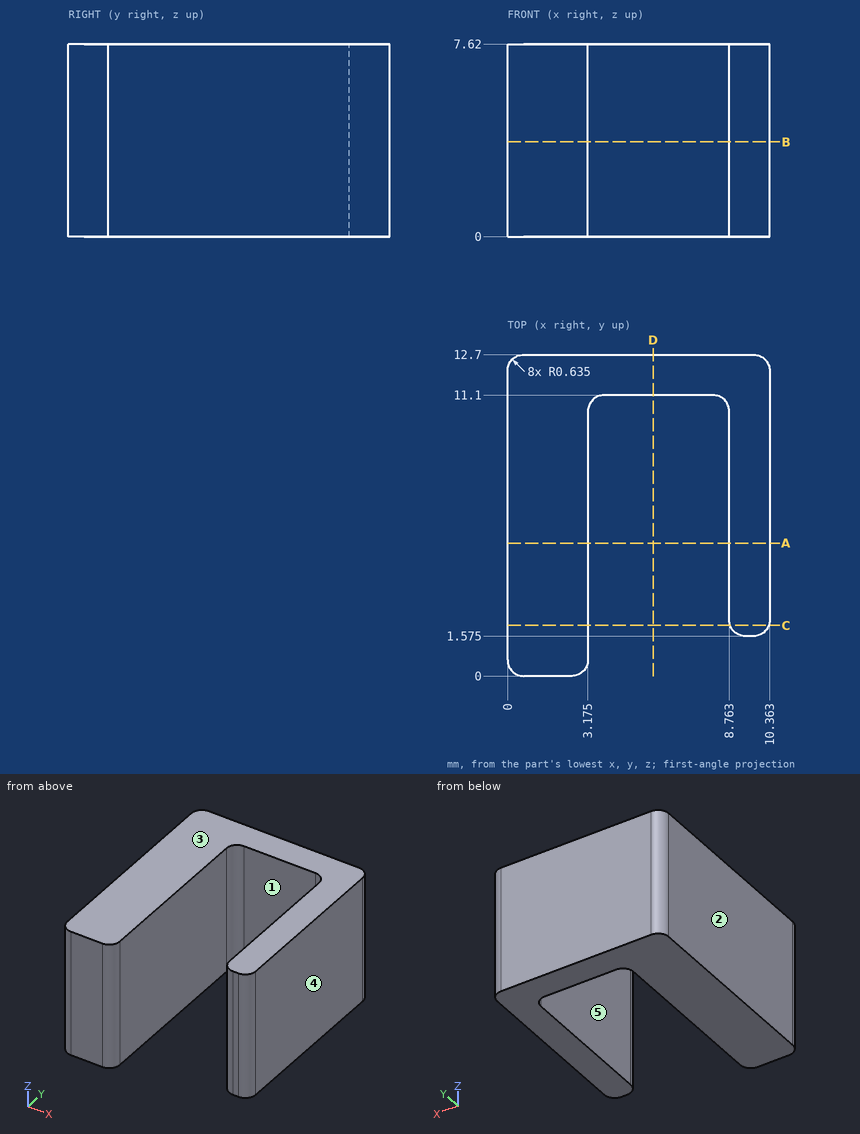
The figure shows three views and two pictorial views of one solid part (mm, origin at its lowest corner). Answer the questions. A direction names the side the tool comes from. Coordinates: 2 decimals unless noted, no trailing zeros. Loops run counter-clockwise (first coordinate to the right, second up) from the corner with the lowest first, then second, coordinate; pieces in that order, holes last.
1) A flat-ended cylindrical pin translates along its axis: pin 1 Ø1.3 at (x, z) = (5.5, 4) entering from -Y. Find the tip coordinate at first contact, or state that the pin passes through.
2) Determine the mould class of the marked faces 1, 2 and 3 for opening direction X: pulls with the +X half, pulls with the -X half, needs draft (parallel to the pull), parting line crosses it, or undercut.
3) A tool of negligible diameter and unlimited length cuts with its end or side. For the marked faces 4 and 5, from which of +Z, -Z, +X, -X, +Y, -Y can it reach the whole face along a straight path? Write none if from no direction.
4) Find section B-B on z = 3.75. Write down the section's boundary in (x, y) (3 decimals).
5) Find section C-C on y = 2. Write down the section's boundary in (x, z) (3 decimals), then the cut area to 3 significant figures.
6) Find section A-A on y = 5.25. Write down the section's boundary in (x, z) (3 decimals), then the cut area to 3 significant figures.
7) Find section D-D on x = 5.75. Write down the section's boundary in (y, z).
8) Find the intervals of material crossed by L1, parallel to X at y = 9.75, z = 2 (3 decimals); L2, parallel to X at y = 0.75, z = 6 (3 decimals); L3, parallel to Y at x = 5.25, z = 3.25, in increasing order.
Values:
1. pin 1: stops at y = 11.1
2. face 1: undercut
2. face 2: pulls with the -X half
2. face 3: needs draft
3. face 4: +Z, -Z, +X, +Y, -Y
3. face 5: +Z, -Z, -Y
4. outline: (0, 0.635) arc R0.635 ccw to (0.635, 0) - (2.54, 0) arc R0.635 ccw to (3.175, 0.635) - (3.175, 10.465) arc R0.635 cw to (3.81, 11.1) - (8.128, 11.1) arc R0.635 cw to (8.763, 10.465) - (8.763, 2.21) arc R0.635 ccw to (9.398, 1.575) - (9.728, 1.575) arc R0.635 ccw to (10.363, 2.21) - (10.363, 12.065) arc R0.635 ccw to (9.728, 12.7) - (0.635, 12.7) arc R0.635 ccw to (0, 12.065) - close
5. outline: (0, 0) - (3.175, 0) - (3.175, 7.62) - (0, 7.62) - close; (8.799, 0) - (10.327, 0) - (10.327, 7.62) - (8.799, 7.62) - close
5. area: 35.8 mm2
6. outline: (0, 0) - (3.175, 0) - (3.175, 7.62) - (0, 7.62) - close; (8.763, 0) - (10.363, 0) - (10.363, 7.62) - (8.763, 7.62) - close
6. area: 36.4 mm2
7. outline: (11.1, 0) - (12.7, 0) - (12.7, 7.62) - (11.1, 7.62) - close
8. L1: x = 0 to 3.175, 8.763 to 10.363
8. L2: x = 0 to 3.175
8. L3: y = 11.1 to 12.7
